Verification items for the finished model (mm, model axes). Give positions to 0.01 mm unless a question says otherwise; leave off trailing zeros. Write each loop counter-clockwise with the first axis right and the second up, starting at its lowest first coordinate (ties: lowest second). Pieces come first, ordered by that corner, then holes. Notation, with made-up numbers: M 22.25,53.5 L 59.25,53.5 A21 ccw 59.25,70.5 Z; hole C 88,20.25 d11. An arc over 180 degrees is marked long. Write item = value, one per line.
Autodesk Fusion 360 part; units mm, degrees
sketch "Sketch1" plane through (0, 0, 0) normal (0, 0, 1) x (1, 0, 0)
  line L0 (203.2, 76.2) -> (-203.2, 76.2)
  line L1 (-203.2, 76.2) -> (-203.2, -76.2)
  line L2 (-203.2, -76.2) -> (203.2, -76.2)
  line L3 (203.2, -76.2) -> (203.2, 76.2)
  line L4 (203.2, 76.2) -> (-203.2, -76.2) construction
  line L5 (-203.2, 76.2) -> (203.2, -76.2) construction
  dimension "d1" = 406.4
  dimension "d2" = 152.4
extrude "Extrude1" add sketch "Sketch1" along normal blind 3.175
sketch "Sketch2" plane through (0, 0, 3.175) normal (0, 0, 1) x (-1, 0, 0)
  line L0 (-203.2, 76.2) -> (-203.2, -76.2)
  line L1 (-203.2, -76.2) -> (203.2, -76.2)
  line L2 (203.2, -76.2) -> (203.2, 76.2)
  line L3 (203.2, 76.2) -> (-203.2, 76.2)
  circle A0 centre (162.56, -44.45) radius 7.9375
  circle A1 centre (111.76, -44.45) radius 7.9375
  circle A2 centre (60.96, -44.45) radius 7.9375
  line L4 (203.2, -44.45) -> (-203.2, -44.45) construction
  line L5 (203.2, -60.325) -> (-203.2, -60.325) construction
  circle A3 centre (162.56, -44.45) radius 10.795 construction
  line L6 (172.6056, -60.325) -> (-27.8584, -60.325) construction
  line L7 (-27.8584, -60.325) -> (-27.8584, -69.85) construction
  line L8 (-27.8584, -69.85) -> (172.6056, -69.85) construction
  line L9 (172.6056, -69.85) -> (172.6056, -60.325) construction
  circle A4 centre (162.56, 0) radius 7.9375
  circle A5 centre (111.76, 0) radius 7.9375
  circle A6 centre (60.96, 0) radius 7.9375
  line L10 (203.2, 0) -> (-203.2, 0) construction
  line L11 (203.2, -15.875) -> (-203.2, -15.875) construction
  line L12 (203.2, 44.45) -> (-203.2, 44.45) construction
  line L13 (203.2, 28.575) -> (-203.2, 28.575) construction
  circle A7 centre (111.76, 44.45) radius 7.9375
  line L14 (183.6475, -15.875) -> (19.338, -15.875) construction
  line L15 (19.338, -15.875) -> (19.338, -25.4) construction
  line L16 (19.338, -25.4) -> (183.6475, -25.4) construction
  line L17 (183.6475, -25.4) -> (183.6475, -15.875) construction
  line L18 (128.4518, 28.575) -> (89.2673, 28.575) construction
  line L19 (89.2673, 28.575) -> (89.2673, 19.05) construction
  line L20 (89.2673, 19.05) -> (128.4518, 19.05) construction
  line L21 (128.4518, 19.05) -> (128.4518, 28.575) construction
  dimension "button" = 15.875
  dimension "d6" = 15.875
  dimension "d7" = 15.875
  dimension "d9" = 50.8
  dimension "d10" = 50.8
  dimension "d12" = 15.875
  dimension "d13" = 21.59
  dimension "d14" = 9.525
  dimension "d17" = 9.525
  dimension "d22" = 15.875
  dimension "d23" = 15.875
  dimension "d24" = 15.875
  dimension "d25" = 50.8
  dimension "d26" = 50.8
  dimension "d28" = 44.45
  dimension "d29" = 15.875
  dimension "d36" = 44.45
  dimension "d37" = 15.875
  dimension "d38" = 15.875
  dimension "d84" = 50.8
  dimension "d85" = 60.96
  dimension "d86" = 60.96
  dimension "d88" = 152.4
  dimension "d89" = 406.4
  dimension "d96" = 10.0456
  dimension "d105" = 9.525
  dimension "d106" = 9.525
  dimension "d107" = 9.525
  dimension "d108" = 9.525
extrude "Extrude3" cut sketch "Sketch2" against normal blind 50.8 contours A0 | A1 | A2 | A4 | A5 | A6 | A7
sketch "Sketch3" plane through (0, 0, 3.175) normal (0, 0, 1) x (-1, 0, 0)
  circle A0 centre (111.76, 0) radius 7.9375
  circle A1 centre (162.56, -44.45) radius 7.9375
  circle A2 centre (60.96, 0) radius 7.9375
  circle A3 centre (162.56, 0) radius 7.9375
  circle A4 centre (111.76, -44.45) radius 7.9375
  circle A5 centre (60.96, -44.45) radius 7.9375
  circle A6 centre (111.76, 44.45) radius 7.9375
  line L0 (-203.2, 76.2) -> (-203.2, -76.2)
  line L1 (-203.2, -76.2) -> (203.2, -76.2)
  line L2 (203.2, -76.2) -> (203.2, 76.2)
  line L3 (203.2, 76.2) -> (-203.2, 76.2)
  circle A7 centre (-92.71, -44.45) radius 7.9375
  circle A8 centre (-92.71, 19.05) radius 7.9375
  circle A9 centre (-60.96, -12.7) radius 7.9375
  circle A10 centre (-124.46, -12.7) radius 7.9375
  line L4 (-92.71, -44.45) -> (-92.71, 19.05) construction
  line L5 (-60.96, -12.7) -> (-124.46, -12.7) construction
  line L6 (-72.6401, -60.325) -> (-119.2488, -60.325) construction
  line L7 (-87.0646, -60.325) -> (-106.5413, -60.325) construction
  line L8 (-106.5413, -60.325) -> (-106.5413, -69.85) construction
  line L9 (-106.5413, -69.85) -> (-87.0646, -69.85) construction
  line L10 (-87.0646, -69.85) -> (-87.0646, -60.325) construction
  line L11 (-84.0964, 3.175) -> (-85.2577, 3.175)
  line L12 (-85.2577, 3.175) -> (-106.3727, 3.175) construction
  line L13 (-86.9218, 3.175) -> (-101.4306, 3.175) construction
  line L14 (-101.4306, 3.175) -> (-101.4306, -6.35) construction
  line L15 (-101.4306, -6.35) -> (-86.9218, -6.35) construction
  line L16 (-86.9218, -6.35) -> (-86.9218, 3.175) construction
  line L17 (-50.0842, -28.575) -> (-73.0383, -28.575) construction
  line L18 (-55.7529, -28.575) -> (-69.6326, -28.575) construction
  line L19 (-69.6326, -28.575) -> (-69.6326, -38.1) construction
  line L20 (-69.6326, -38.1) -> (-55.7529, -38.1) construction
  line L21 (-55.7529, -38.1) -> (-55.7529, -28.575) construction
  line L22 (-117.6854, -28.575) -> (-146.3556, -28.575) construction
  line L23 (-119.2474, -28.575) -> (-139.2811, -28.575) construction
  line L24 (-139.2811, -28.575) -> (-139.2811, -38.1) construction
  line L25 (-139.2811, -38.1) -> (-119.2474, -38.1) construction
  line L26 (-119.2474, -38.1) -> (-119.2474, -28.575) construction
  line L27 (-156.21, -44.45) -> (-156.21, 19.05) construction
  circle A11 centre (-156.21, -44.45) radius 7.9375
  circle A12 centre (-156.21, 19.05) radius 7.9375
  line L28 (-162.1579, 3.175) -> (-182.2496, 3.175) construction
  line L29 (-156.3761, -60.325) -> (-181.7712, -60.325) construction
  line L30 (-151.6704, -60.325) -> (-180.3361, -60.325) construction
  line L31 (-180.3361, -60.325) -> (-180.3361, -69.85) construction
  line L32 (-180.3361, -69.85) -> (-151.6704, -69.85) construction
  line L33 (-151.6704, -69.85) -> (-151.6704, -60.325) construction
  line L34 (-151.7847, 3.175) -> (-164.1052, 3.175) construction
  line L35 (-164.1052, 3.175) -> (-164.1052, -6.35) construction
  line L36 (-164.1052, -6.35) -> (-151.7847, -6.35) construction
  line L37 (-151.7847, -6.35) -> (-151.7847, 3.175) construction
  circle A13 centre (60.96, 0) radius 7.9375
  line L38 (-92.71, -44.45) -> (-92.71, -63.514) construction
  circle A14 centre (31.75, 57.15) radius 7.9375
  circle A15 centre (-31.75, 57.15) radius 7.9375
  line L39 (-19.4302, 41.275) -> (-47.0824, 41.275) construction
  line L40 (-18.4863, 41.275) -> (-133.9128, 41.275) construction
  line L41 (46.0464, 41.275) -> (2.2756, 41.275) construction
  line L42 (2.2756, 41.275) -> (2.2756, 34.925) construction
  line L43 (2.2756, 34.925) -> (46.0464, 34.925) construction
  line L44 (46.0464, 34.925) -> (46.0464, 41.275) construction
  line L45 (-18.4863, 41.275) -> (-69.5814, 41.3535) construction
  line L46 (-69.5814, 41.3535) -> (-69.5912, 35.0035) construction
  line L47 (-69.5912, 35.0035) -> (-18.496, 34.925) construction
  line L48 (-18.496, 34.925) -> (-18.4863, 41.275) construction
  circle A16 centre (-95.25, 57.15) radius 7.9375
  circle A17 centre (-158.75, 57.15) radius 7.9375
  line L49 (-86.5667, 41.275) -> (-118.397, 41.2226) construction
  line L50 (-118.397, 41.2226) -> (-118.3865, 34.8727) construction
  line L51 (-118.3865, 34.8727) -> (-86.5562, 34.925) construction
  line L52 (-86.5562, 34.925) -> (-86.5667, 41.275) construction
  line L53 (-148.8254, 41.4006) -> (-186.2835, 41.4006) construction
  line L54 (-186.2835, 41.4006) -> (-186.2835, 34.6904) construction
  line L55 (-186.2835, 34.6904) -> (-148.8254, 34.6904) construction
  line L56 (-148.8254, 34.6904) -> (-148.8254, 41.4006) construction
  point P0 (-92.71, -12.7)
  point P1 (-156.21, -12.7)
  dimension "d46" = 15.875
  dimension "d47" = 15.875
  dimension "d48" = 15.875
  dimension "d49" = 15.875
  dimension "d52" = 63.5
  dimension "d56" = 15.875
  dimension "d57" = 9.525
  dimension "d58" = 9.525
  dimension "d59" = 15.875
  dimension "d60" = 9.525
  dimension "d61" = 9.525
  dimension "d62" = 15.875
  dimension "d63" = 9.525
  dimension "d64" = 9.525
  dimension "d65" = 15.875
  dimension "d66" = 9.525
  dimension "d67" = 9.525
  dimension "d71" = 15.875
  dimension "d72" = 15.875
  dimension "d73" = 9.525
  dimension "d74" = 9.525
  dimension "d75" = 15.875
  dimension "d76" = 15.875
  dimension "d77" = 9.525
  dimension "d78" = 9.525
  dimension "d98" = 63.5
  dimension "d99" = 63.5
  dimension "d100" = 31.75
  dimension "d101" = 31.75
  dimension "d102" = 31.75
  dimension "d103" = 31.75
  dimension "d104" = 406.4
  dimension "d109" = 60.96
  dimension "d110" = 63.5
  dimension "d111" = 38.1
  dimension "d112" = 15.875
  dimension "d113" = 15.875
  dimension "d114" = 6.35
  dimension "d115" = 15.875
  dimension "d116" = 6.35
  dimension "d117" = 15.875
  dimension "d118" = 6.35
  dimension "d119" = 6.35
  dimension "d120" = 31.75
  dimension "d121" = 15.875
  dimension "d122" = 15.875
  dimension "d123" = 63.5
  dimension "d124" = 63.5
  dimension "d125" = 6.35
  dimension "d126" = 6.35
  dimension "d127" = 6.35
extrude "Extrude4" cut sketch "Sketch3" against normal blind 27.94 contours A7 | A8 | A9 | A10 | A11 | A12 | A14 | A15 | A16 | A17
sketch "Sketch4" plane through (0, 0, 3.175) normal (0, 0, 1) x (-1, 0, 0)
equation "d7 = d6"
equation "d9 = d25"
equation "d10 = d25"
equation "d22 = d6"
equation "d23 = d6"
equation "d24 = d6"
equation "d26 = d25"
equation "d38 = d6"
equation "d46 = d6"
equation "d47 = d6"
equation "d48 = d6"
equation "d49 = d6"
equation "d61 = d78"
equation "d64 = d78"
equation "d71 = d6"
equation "d72 = d6"
equation "d84 = d25"
equation "d85 = d89 * 0.15"
equation "d86 = d85"
equation "d99 = d98"
equation "d100 = d98 / 2"
equation "d101 = d100"
equation "d102 = d100"
equation "d103 = d100"
equation "d109 = d104 * 0.15"
equation "d110 = d98"
equation "d111 = d101 + 0.25 in"
equation "d112 = d47"
equation "d113 = d47"
equation "d115 = d62"
equation "d117 = d115"
equation "d120 = d110 / 2"
equation "d121 = d113"
equation "d122 = d113"
equation "d123 = d110"
equation "d124 = d99"
1) Draft check along X on faces 1 (the flat face through (-3, 1, 3.175)), 2 (the cylindrical face through (27.48, -63.84, 1.61)). Enter one of: +X half, -X half, draft (parallel to the pull), parting line (faces both ways), or undercut.
From the geometry:
face_1 = draft
face_2 = undercut
2) Cross-section at A-A on y = 0. Record the boundary of the cut face in (x, z) (1 decimal), plus the area to 3 significant figures.
From the geometry:
outline = M -203.2,0 L -170.5,0 L -170.5,3.2 L -203.2,3.2 Z; M -154.6,0 L -119.7,0 L -119.7,3.2 L -154.6,3.2 Z; M -103.8,0 L -68.9,0 L -68.9,3.2 L -103.8,3.2 Z; M -53,0 L 203.2,0 L 203.2,3.2 L -53,3.2 Z
area = 1,140 mm^2
3) Depth check by flat-ended pin: P1, Ø14.5, axis at x = 156.21, y = -19.05, coming from the +Z side. Enter the tip coordinate at first touch or a pass-through.
From the geometry:
P1 = through
4) Cross-section at C-C on x = -111.76. Record the boundary of the cut face in (y, z) (1 decimal), plus the area to 3 significant figures.
From the geometry:
outline = M -76.2,0 L -52.4,0 L -52.4,3.2 L -76.2,3.2 Z; M -36.5,0 L -7.9,0 L -7.9,3.2 L -36.5,3.2 Z; M 7.9,0 L 36.5,0 L 36.5,3.2 L 7.9,3.2 Z; M 52.4,0 L 76.2,0 L 76.2,3.2 L 52.4,3.2 Z
area = 333 mm^2
5) Material ranges on probe 1 along X at (y, z) = (-57.15, 1.85); probe 2 along X at (y, z) = (0, 1.15); probe 3 along Y at (x, z) = (-111.76, 1.7), recorded low to high. Write a range as from..to.
From the geometry:
probe_1 = -203.2..-39.69, -23.81..23.81, 39.69..87.31, 103.19..150.81, 166.69..203.2
probe_2 = -203.2..-170.5, -154.62..-119.7, -103.82..-68.9, -53.02..203.2
probe_3 = -76.2..-52.39, -36.51..-7.94, 7.94..36.51, 52.39..76.2
6) Cross-section at B-B on z = 1.8. Count the separate pieces of the cut face and the enclosed holes in it, plus the area to 3 significant figures.
From the geometry:
separate_pieces = 1
enclosed_holes = 17
area = 58,600 mm^2
7) Cross-section at D-D on y = -19.05. Record the boundary of the cut face in (x, z) (1 decimal).
From the geometry:
outline = M -203.2,0 L 84.8,0 L 84.8,3.2 L -203.2,3.2 Z; M 100.6,0 L 148.3,0 L 148.3,3.2 L 100.6,3.2 Z; M 164.1,0 L 203.2,0 L 203.2,3.2 L 164.1,3.2 Z
